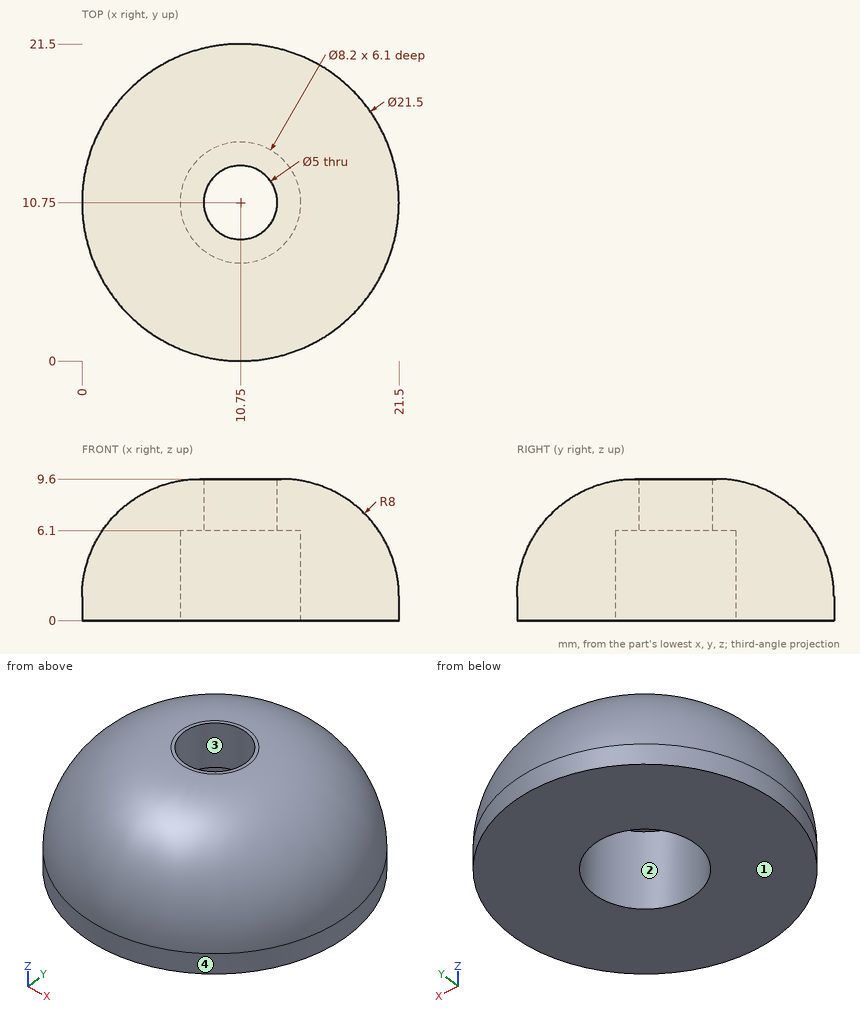
Source: three-view drawing plus pictorial views. Frame: mm from the lowest corner of the part. Give positions to 0.01 mm unless a question says otherwise; leave off trailing zeros. Put each result on its own line as item: value.
Item 1: Draft query along X for the marked faces 1, 2, 3 and 4. Return one class per face: +X half, -X half, draft (parallel to the pull), parting line (faces both ways), or undercut.
Found:
face 1: draft
face 2: undercut
face 3: undercut
face 4: parting line
Item 2: Contact query for flat-ended pins moving along their axis: pin 1 (3 mm diameter, centred on x = 11.5, z = 3, fed in from -Y); pin 2 (4 mm diameter, centred on x = 11.5, y = 9.5, fed in from -Z); pin 3 (2 mm diameter, centred on x = 18.5, y = 13.5, fed in from +Z); pin 4 (3 mm diameter, centred on x = 10.75, y = 10.75, fed in from -Z). Output: stop coordinate, or through.
Found:
pin 1: stops at y = 0
pin 2: stops at z = 6.1
pin 3: stops at z = 8.23
pin 4: passes through
Item 3: Ray query, L1, parallel to Y at x = 10.75, z = 2.25; L2, parallel to Y at x = 7, z = 2.5; L3, parallel to X at y = 7, z = 2.75. Return the intervals inside material, ascending. Write a range as from..to.
Found:
L1: y = 0.03..6.65, 14.85..21.47
L2: y = 0.73..9.09, 12.41..20.77
L3: x = 0.76..9.09, 12.41..20.74
